```python
from build123d import *

# Parameters (mm, degrees)
SKETCH1_W                  = 63
SKETCH1_H                  = 24
BOSS_EXTRUDE1_DEPTH        = 20
SKETCH2_W                  = 15
SKETCH2_H                  = 15
CUT_EXTRUDE1_DEPTH         = 59.326666286
SKETCH3_W                  = 49
SKETCH3_H                  = 7
BOSS_EXTRUDE2_DEPTH        = 10
SKETCH4_W                  = 49
SKETCH4_H                  = 7
BOSS_EXTRUDE3_DEPTH        = 10
HOLE1_D                    = 18
HOLE1_DEPTH                = 15
F_6_CLEARANCE_HOLE1_D      = 4.2
F_6_CLEARANCE_HOLE1_DEPTH  = 7
F_6_CLEARANCE_HOLE2_D      = 4.2
F_6_CLEARANCE_HOLE2_DEPTH  = 7
F_10_CLEARANCE_HOLE1_D     = 5.5
F_10_CLEARANCE_HOLE1_DEPTH = 24
F_10_CLEARANCE_HOLE2_D     = 5.5
F_10_CLEARANCE_HOLE2_DEPTH = 7
CHAMFER1_SIZE              = 0.4
FILLET1_R                  = 4
FILLET2_R                  = 7
BOSS_EXTRUDE5_START        = 2.54
SKETCH20_R                 = 9
BOSS_EXTRUDE5_DEPTH        = 2.54
SKETCH21_R                 = 3.2639
CUT_EXTRUDE4_DEPTH         = 60.030937651


with BuildPart() as part:
    # Sketch1 → Boss-Extrude1 (new body)
    with BuildSketch(Plane.XY.offset(5)):
        with Locations((19.5, 0)):
            Rectangle(SKETCH1_W, SKETCH1_H)
    extrude(amount=-BOSS_EXTRUDE1_DEPTH)

    # Sketch2 → Cut-Extrude1 (cut, through all)
    with BuildSketch(Plane.XZ.offset(12)):
        with Locations((19.5, -7.5)):
            Rectangle(SKETCH2_W, SKETCH2_H)
    extrude(amount=-CUT_EXTRUDE1_DEPTH, mode=Mode.SUBTRACT)

    # Sketch3 → Boss-Extrude2 (add)
    with BuildSketch(Plane.XY.offset(5)):
        with Locations((19.5, -8.5)):
            Rectangle(SKETCH3_W, SKETCH3_H)
    extrude(amount=BOSS_EXTRUDE2_DEPTH)

    # Sketch4 → Boss-Extrude3 (add)
    with BuildSketch(Plane.XY.offset(5)):
        with Locations((19.5, 8.5)):
            Rectangle(SKETCH4_W, SKETCH4_H)
    extrude(amount=BOSS_EXTRUDE3_DEPTH)

    # Hole1
    with Locations(Plane(origin=(0, 0, -15), x_dir=(-1, 0, 0), z_dir=(0, 0, -1))):
        with Locations((0, 0), (-39, 0)):
            Hole(HOLE1_D / 2, depth=HOLE1_DEPTH)

    # #6 Clearance Hole1
    with Locations(Plane(origin=(0, 5, 0), x_dir=(-1, 0, 0), z_dir=(0, -1, 0))):
        with Locations((-0.75, -10)):
            Hole(F_6_CLEARANCE_HOLE1_D / 2, depth=F_6_CLEARANCE_HOLE1_DEPTH)

    # #6 Clearance Hole2
    with Locations(Plane(origin=(0, 12, 0), x_dir=(1, 0, 0), z_dir=(0, 1, 0))):
        with Locations((38.25, -10), (25.75, -10), (13.25, -10)):
            Hole(F_6_CLEARANCE_HOLE2_D / 2, depth=F_6_CLEARANCE_HOLE2_DEPTH)

    # #10 Clearance Hole1
    with Locations(Plane(origin=(0, -12, 0), x_dir=(-1, 0, 0), z_dir=(0, -1, 0))):
        with Locations((-13.25, -10), (-0.75, -10)):
            Hole(F_10_CLEARANCE_HOLE1_D / 2, depth=F_10_CLEARANCE_HOLE1_DEPTH)

    # #10 Clearance Hole2
    with Locations(Plane(origin=(0, -5, 0), x_dir=(1, 0, 0), z_dir=(0, 1, 0))):
        with Locations((38.25, -10), (25.75, -10)):
            Hole(F_10_CLEARANCE_HOLE2_D / 2, depth=F_10_CLEARANCE_HOLE2_DEPTH)

    # Chamfer1
    chamfer1_edges = [part.edges().sort_by_distance(p)[0] for p in [
        (10.5, 12, 10),
        (10.5, -12, 10),
        (28.5, -12, 10),
        (41, -12, 10),
        (27.85, 12, 10),
        (40.35, 12, 10),
        (-2, 12, 10),
        (-2, -12, 10),
    ]]
    chamfer(chamfer1_edges, length=CHAMFER1_SIZE)

    # Fillet1
    fillet1_edges = [part.edges().sort_by_distance(p)[0] for p in [
        (12, 12, -7.5),
        (27, 12, -7.5),
        (12, -12, -7.5),
        (27, -12, -7.5),
    ]]
    fillet(fillet1_edges, radius=FILLET1_R)

    # Fillet2
    fillet2_edges = [part.edges().sort_by_distance(p)[0] for p in [
        (51, -12, -5),
        (-12, 12, -5),
        (51, 12, -5),
        (-12, -12, -5),
    ]]
    fillet(fillet2_edges, radius=FILLET2_R)

    # Sketch20 → Boss-Extrude5 (add)
    # profile 1 of 2: a face of its own
    with BuildSketch(Plane(origin=(0, 0, -15), x_dir=(-1, 0, 0), z_dir=(0, 0, -1)).offset(BOSS_EXTRUDE5_START)):
        with BuildLine():
            Line((12, -5), (12, 5))
            ThreePointArc((12, 5), (9.949747468, 9.949747468), (5, 12))
            Line((5, 12), (-8, 12))
            ThreePointArc((-8, 12), (-10.828427125, 10.828427125), (-12, 8))
            Line((-12, 8), (-12, -8))
            ThreePointArc((-12, -8), (-10.828427125, -10.828427125), (-8, -12))
            Line((-8, -12), (5, -12))
            ThreePointArc((5, -12), (9.949747468, -9.949747468), (12, -5))
        make_face()
        Circle(SKETCH20_R, mode=Mode.SUBTRACT)
    # profile 2 of 2: a face of its own
    with BuildSketch(Plane(origin=(0, 0, -15), x_dir=(-1, 0, 0), z_dir=(0, 0, -1)).offset(BOSS_EXTRUDE5_START)):
        with BuildLine():
            Line((-51, 5), (-51, -5))
            ThreePointArc((-51, -5), (-48.949747468, -9.949747468), (-44, -12))
            Line((-44, -12), (-31, -12))
            ThreePointArc((-31, -12), (-28.171572875, -10.828427125), (-27, -8))
            Line((-27, -8), (-27, 8))
            ThreePointArc((-27, 8), (-28.171572875, 10.828427125), (-31, 12))
            Line((-31, 12), (-44, 12))
            ThreePointArc((-44, 12), (-48.949747468, 9.949747468), (-51, 5))
        make_face()
        with Locations((-39, 0)):
            Circle(SKETCH20_R, mode=Mode.SUBTRACT)
    extrude(amount=-BOSS_EXTRUDE5_DEPTH)

    # Sketch21 → Cut-Extrude4 (cut, through all)
    with BuildSketch(Plane(origin=(0, 12, 0), x_dir=(1, 0, 0), z_dir=(0, 1, 0))):
        with Locations(Location((37.5, 8.89, 0), (0, 0, 270))):
            Circle(SKETCH21_R)
        with Locations(Location((1.5, 8.89, 0), (0, 0, 270))):
            Circle(SKETCH21_R)
    extrude(amount=-CUT_EXTRUDE4_DEPTH, mode=Mode.SUBTRACT)


solid = part.part
```
Geometry: final body of the model. Coordinates: model frame, mm. A direction names the side the tool comes from. Coordinates: 2 decimals unless noted, no trailing zeros. Order: outer loops, then holes, each group sorted by start corner. A loop starts at its lowest first (then second) coordinate and runs counter-clockwise, first axis right, second up. Notation, with made-up numbers: (19.5, 67.25) - (64.5, 67.25) arc R20 cw to (64.5, 98.25) - close; hole circle Ø1 at (34.5, 38). An arc over 180 degrees is marked (long way). Write each question's results on one line, items separated by ' | '.
1) Section B-B, the plane z = -1.5. Return loops of the section in (x, y).
Results list:
outline: (-12, -5) arc R7 ccw to (-5, -12) - (8, -12) arc R4 ccw to (12, -8) - (12, 8) arc R4 ccw to (8, 12) - (-5, 12) arc R7 ccw to (-12, 5) - close; (27, -8) arc R4 ccw to (31, -12) - (44, -12) arc R7 ccw to (51, -5) - (51, 5) arc R7 ccw to (44, 12) - (31, 12) arc R4 ccw to (27, 8) - close; hole circle Ø18 at (0, 0); hole circle Ø18 at (39, 0)
2) Line query: line 1 (X direction, y = -9.25, z = 10); line 2 (X direction, y = 10.25, z = 10); line 3 (Z direction, x = 0.75, y = -8). Output: solid intervals per line, ascending. Write a range as from..to.
Results list:
line 1: -5..-2, 3.5..10.5, 16..23, 28.5..35.5, 41..44 | line 2: -5..-2, 3.5..10.5, 16..23.65, 27.85..36.15, 40.35..44 | line 3: 0..7.25, 12.75..15
3) Pin query (flat end, axial travel): pin 1 (5 mm diameter, centred on y = 4.5, z = 11, fed in from -X). Return the tip coordinate at first contact, or that it passes through.
Results list:
pin 1: x = -5
4) Pull-direction query (Y, two-part tool) for faces 4 (the flat face through (20, -12, 2)), 5 (the flat face through (19, -5, 10)), 6 (the flat face through (6, -8, -17.54)); classes: pulls with the +Y half, pulls with the -Y half, needs draft (parallel to the pull), parting line crosses it, or undercut.
Results list:
face 4: pulls with the -Y half | face 5: undercut | face 6: needs draft
5) Section D-D, the plane z = -8.89. State how many separate pieces and enclosed holes the cut face has, plus the area to 3 significant figures.
Results list:
separate pieces: 4 | enclosed holes: 0 | area: 500 mm^2
6) Section C-C, the plane y = 0. Return loops of the section in (x, z), plus the area to 3 significant figures.
Results list:
outline: (-12, -17.54) - (-9, -17.54) - (-9, 0) - (9, 0) - (9, -17.54) - (12, -17.54) - (12, 0) - (27, 0) - (27, -17.54) - (30, -17.54) - (30, 0) - (48, 0) - (48, -17.54) - (51, -17.54) - (51, 5) - (-12, 5) - close | area: 525 mm^2
7) Section A-A, the plane x = 13.25. Return loops of the section in (y, z).
Results list:
outline: (-12, 0) - (12, 0) - (12, 6.85) - (11.6, 7.25) - (5, 7.25) - (5, 5) - (-5, 5) - (-5, 7.25) - (-11.6, 7.25) - (-12, 6.85) - close; (-12, 13.15) - (-11.6, 12.75) - (-5, 12.75) - (-5, 15) - (-12, 15) - close; (5, 12.75) - (11.6, 12.75) - (12, 13.15) - (12, 15) - (5, 15) - close
8) Set-up query: faces 1 (the cylindrical face through (28.5, -8.3, 9.9)), 2 (the cylindrical face through (4.736, 10.333, -9.315)), 3 (the flat face through (27, 0, -9)). Return all of +Z, -Z, +X, -X, +Y, -Y with unobstructed straight access to the full face (end or side cutting, diameter ignored); none if empty.
Results list:
face 1: -Y | face 2: +Y, -Y | face 3: -Z, +Y, -Y
